Read the model definition and answer for the solid it produces. Units are mm, in the model's axes. A direction names the side the tool comes from. Coordinates: 2 decimals unless noted, no trailing zeros. Order: outer loops, then holes, each group sorted by start corner. A loop starts at its lowest first (then second) coordinate and runs counter-clockwise, first axis right, second up. Notation, with made-up numbers: (71, 60) - (99, 60) arc R14 ccw to (99, 77) - close; hole circle Ø1 at (73, 20). An arc over 180 degrees is marked (long way). Write item = value, one per line.
from build123d import *

# Parameters (mm, degrees)
ESBO_O1_R                = 59.5
RESSALTO_EXTRUS_O1_DEPTH = 55
ESBO_O2_R                = 50.8
CORTE_EXTRUS_O1_DEPTH    = 45
ESBO_O3_R                = 59.5
ESBO_O3_R_2              = 56.5
CORTE_EXTRUS_O2_DEPTH    = 45


with BuildPart() as part:
    # Esboço1 → Ressalto-extrusão1 (new body)
    with BuildSketch(Plane(origin=(0, 0, 0), x_dir=(1, 0, 0), z_dir=(0, 1, 0))):
        Circle(ESBO_O1_R)
    extrude(amount=RESSALTO_EXTRUS_O1_DEPTH)

    # Esboço2 → Corte-extrusão1 (cut)
    with BuildSketch(Plane(origin=(0, 55, 0), x_dir=(1, 0, 0), z_dir=(0, 1, 0))):
        Circle(ESBO_O2_R)
    extrude(amount=-CORTE_EXTRUS_O1_DEPTH, mode=Mode.SUBTRACT)

    # Esboço3 → Corte-extrusão2 (cut)
    with BuildSketch(Plane(origin=(0, 55, 0), x_dir=(1, 0, 0), z_dir=(0, 1, 0))):
        Circle(ESBO_O3_R)
        Circle(ESBO_O3_R_2, mode=Mode.SUBTRACT)
    extrude(amount=-CORTE_EXTRUS_O2_DEPTH, mode=Mode.SUBTRACT)


solid = part.part
1) The part is cut by section C-C (y = 17). Determine the outline of the cut face in (x, z), and give its area (3 significant figures).
Returned:
outline = circle Ø113 at (0, 0); hole circle Ø101.6 at (0, 0)
area = 1,920 mm^2
2) Determine the mould class of faces 3 (the face through (-1, 10, -1)), 4 (the face through (53, 10, 22)), 5 (the face through (31.99, 4.93, -50.17)) for opening direction X: pulls with the +X half, pulls with the -X half, needs draft (parallel to the pull), parting line crosses it, or undercut.
Returned:
face_3 = undercut
face_4 = needs draft
face_5 = parting line crosses it
3) The part is cut by section B-B (x = 39). Determine the outline of the cut face in (y, z).
Returned:
outline = (0, -44.94) - (10, -44.94) - (10, -40.88) - (55, -40.88) - (55, -32.55) - (10, -32.55) - (10, 32.55) - (55, 32.55) - (55, 40.88) - (10, 40.88) - (10, 44.94) - (0, 44.94) - close
4) Flat-ended cylindrical pins translate along their axes: pin 1 Ø3 at (x, z) = (-37, 17) entering from +Y; pin 2 Ø12 at (x, z) = (0, -4) entering from -Y; pin 3 Ø8 at (x, y) = (30.5, 25.5) entering from +Z; pin 4 Ø8 at (x, y) = (-47, 8) entering from -Z. Find the tip coordinate at first contact, or state that the pin passes through.
Returned:
pin_1 = 10
pin_2 = 0
pin_3 = 49.9
pin_4 = -41.12
5) Straight lines are drawn through the part: line 1 along X through (y, z) = (20.5, 0); line 2 along Y through (x, z) = (-29, 23). For each, find the intervals that lie inside material, in ascending order. Write a range as from..to.
Returned:
line_1 = -56.5..-50.8, 50.8..56.5
line_2 = 0..10
6) The part is cut by section A-A (z = 0). Determine the outline of the cut face in (x, y), and give its area (3 significant figures).
Returned:
outline = (-59.5, 0) - (59.5, 0) - (59.5, 10) - (56.5, 10) - (56.5, 55) - (50.8, 55) - (50.8, 10) - (-50.8, 10) - (-50.8, 55) - (-56.5, 55) - (-56.5, 10) - (-59.5, 10) - close
area = 1,700 mm^2
7) For faces 1 (the face through (-11.012, 32.815, 49.592)), 2 (the face through (-1, 0, -1)), determine the directions among +Z, -Z, +X, -X, +Y, -Y from which every point of the face is accessible in a straight line to the end or side of a thin tool.
Returned:
face_1 = +Y
face_2 = +Z, -Z, +X, -X, -Y
